```python
from build123d import *

# Parameters (mm, degrees)
SKETCH001_W  = 30
SKETCH001_H  = 14
PAD_DEPTH    = 7.2
SKETCH002_R  = 0.225
PAD001_DEPTH = 5


with BuildPart() as part:
    # Sketch001 → Pad (new body)
    with BuildSketch(Plane.XY):
        Rectangle(SKETCH001_W, SKETCH001_H)
    extrude(amount=PAD_DEPTH)

    # Sketch002 (on Face6 of Pad) → Pad001 (join)
    with BuildSketch(Plane.XY.offset(7.2)):
        with Locations((-3.81, -5.08)):
            Circle(SKETCH002_R)
        with Locations((-6.35, -5.08)):
            Circle(SKETCH002_R)
        with Locations((-1.27, -5.08)):
            Circle(SKETCH002_R)
        with Locations((1.27, -5.08)):
            Circle(SKETCH002_R)
        with Locations((3.81, -5.08)):
            Circle(SKETCH002_R)
        with Locations((6.35, -5.08)):
            Circle(SKETCH002_R)
        with Locations((-3.81, 5.08)):
            Circle(SKETCH002_R)
        with Locations((-6.35, 5.08)):
            Circle(SKETCH002_R)
        with Locations((-1.27, 5.08)):
            Circle(SKETCH002_R)
        with Locations((1.27, 5.08)):
            Circle(SKETCH002_R)
        with Locations((3.81, 5.08)):
            Circle(SKETCH002_R)
        with Locations((6.35, 5.08)):
            Circle(SKETCH002_R)
    extrude(amount=PAD001_DEPTH)


solid = part.part
```
Work out the finished part from the listing and answer in its coordinate system (mm). Give positions to 0.01 mm unless a question says otherwise; leave off trailing zeros. Order: outer loops, then holes, each group sorted by start corner. A loop starts at its lowest first (then second) coordinate and runs counter-clockwise, first axis right, second up.
1. Each of these flat-tipped pins is pushed along its axis until it touches: P1, Ø5, axis at x = -6.5, y = 1, coming from the +Z side; P2, Ø4, axis at y = 5, z = 10.5, coming from the -X side (3 decimals). Where does it stop, or does it pass through?
Result sheet:
P1: stops at z = 7.2
P2: stops at x = -6.575
2. Section C-C, the plane x = 7.75 is taken. Determine the outline of the cut face in (y, z), and give its area (3 significant figures).
Result sheet:
outline: (-7, 0) - (7, 0) - (7, 7.2) - (-7, 7.2) - close
area: 101 mm2
3. Section B-B, the plane y = 3.5 is taken. Determine the outline of the cut face in (x, z).
Result sheet:
outline: (-15, 0) - (15, 0) - (15, 7.2) - (-15, 7.2) - close
4. Straight lines are drawn through the part: L1, parallel to Z at x = -7, y = -6; L2, parallel to Y at x = 3.75, z = 9. For each, find the intervals that lie inside material, in ascending order.
Result sheet:
L1: z = 0 to 7.2
L2: y = -5.3 to -4.86, 4.86 to 5.3
5. Section A-A, the plane z = 10.25 is taken. Give the number of separate pieces and of enclosed holes in the cut face, and give its area (3 significant figures).
Result sheet:
separate pieces: 12
enclosed holes: 0
area: 1.91 mm2
